Answer from the drawing. Dimensions are ordinates in mm from the lowest x, y and z of the part. A direction names the side the tool comes from. Give positions to 0.01 mm unless a question says otherwise; leave off trailing zeros. Order: outer loops, then holes, each group sorted by start corner. A loop starts at its lowest first (then second) coordinate and runs counter-clockwise, first axis right, second up.
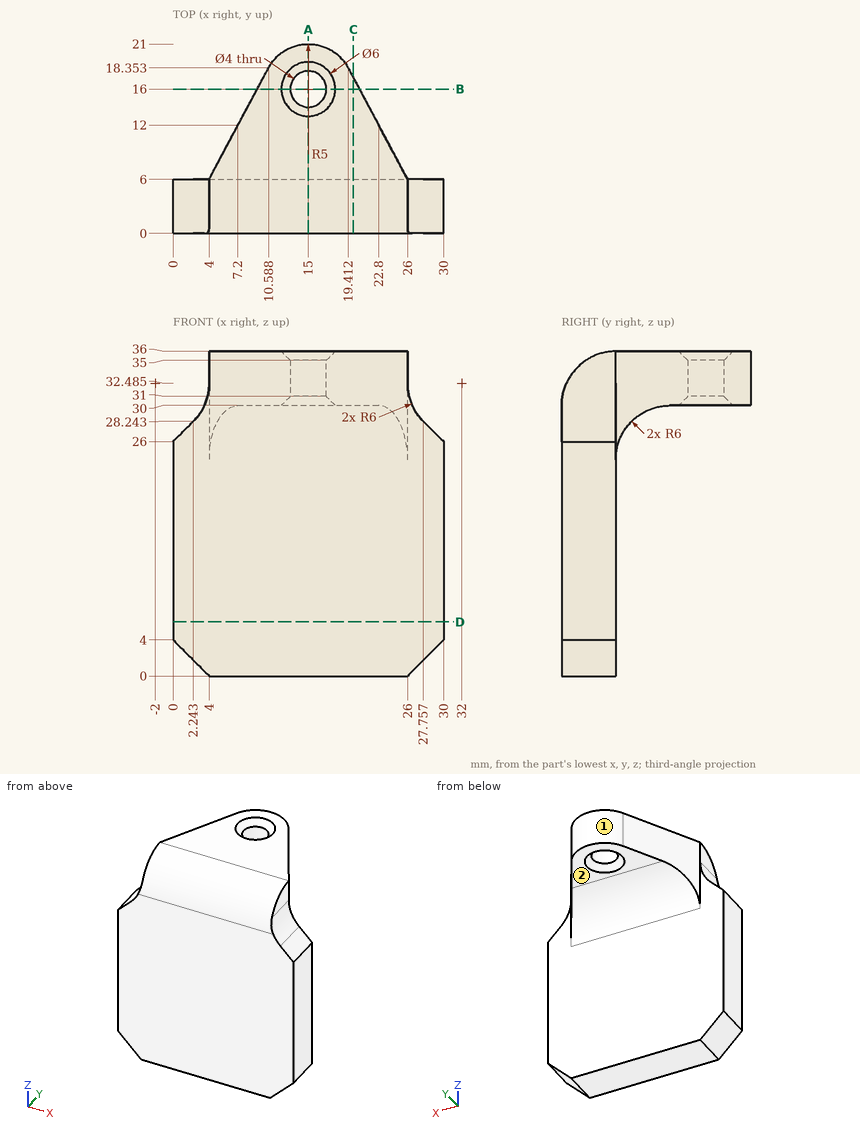
1) Given pin 1 (12 mm diameter, centred on y = 6.5, z = 12, fed in from -X); pin 2 (4 mm diameter, centred on x = 6.5, y = 9.5, fed in from -Z); pin 3 (4 mm diameter, centred on y = 4, z = 35, fed in from +X); pin 4 (15 mm diameter, centred on x = 20, z = 13, fed in from +Y), each flat-ended and moving along its own axis, determine where each tip first touches the part or whether it passes through.
Final values:
pin 1: stops at x = 0
pin 2: stops at z = 27.97
pin 3: stops at x = 26
pin 4: stops at y = 6
2) Consider L1, parallel to Y at x = 6, z = 2; L2, parallel to Z at x = 10.5, y = 16; L3, parallel to Z at x = 22, y = 5.75 (1 decimal). Determine where each line is inside the solid, lowest interval first.
Final values:
L1: y = 0 to 6
L2: z = 30 to 36
L3: z = 0 to 36
3) The part is cut by section B-B on y = 16. Determine the outline of the cut face in (x, z).
Final values:
outline: (9.33, 30) - (12, 30) - (13, 31) - (13, 35) - (12, 36) - (9.33, 36) - close; (17, 31) - (18, 30) - (20.67, 30) - (20.67, 36) - (18, 36) - (17, 35) - close
4) The part is cut by section A-A on x = 15. Determine the outline of the cut face in (y, z).
Final values:
outline: (0, 0) - (6, 0) - (6, 24) arc R6 cw to (12, 30) - (13, 30) - (14, 31) - (14, 35) - (13, 36) - (6, 36) arc R6 ccw to (0, 30) - close; (18, 31) - (19, 30) - (21, 30) - (21, 36) - (19, 36) - (18, 35) - close
5) A tool of negligible diameter and unlimited length cuts with its end or side. For the marked faces 1 and 2, from which of +Z, -Z, +X, -X, +Y, -Y can it reach the whole face along a straight path? Write none if from no direction.
Final values:
face 1: +Z, -Z, +Y
face 2: -Z, +X, -X, +Y
6) The part is cut by section D-D on z = 6. Determine the outline of the cut face in (x, y).
Final values:
outline: (0, 0) - (30, 0) - (30, 6) - (0, 6) - close
7) The part is cut by section C-C on x = 20. Determine the outline of the cut face in (y, z).
Final values:
outline: (0, 0) - (6, 0) - (6, 24) arc R6 cw to (12, 30) - (17.25, 30) - (17.25, 36) - (6, 36) arc R6 ccw to (0, 30) - close
